Could you check a few things on this drawing? It's one solid part, dimensions in mm from its lowest x, y, z. A direction names the side the tool comes from. Coordinates: 2 decimals unless noted, no trailing zeros. Order: outer loops, then holes, each group sorted by start corner. A loop starts at its lowest first (then second) coordinate and runs counter-clockwise, first axis right, second up. Notation, with made-up numbers: M 13,3.5 L 39,3.5 A21 cw 39,28.5 Z; hole C -37.5,-26.5 d4. An arc over 180 degrees is marked long. Answer as CSV lines item,"result". Start each with the question number.
1. If we section it at A-A (z = 7.75): List the corners of the cut face in (x, y) for me, plus the area to 3 significant figures.
2. I need wall thicknesses on line 1 along Z through (x, y) = (9, 3.5); line 2 along Z through (x, y) = (5, 2.6); line 3 along Z through (x, y) = (5, 1.2). Which ranges of each line are inside material? Lowest first, please. Write a range as from..to.
3. If we mould it in two halves opening along Z, with no side actions, what happens to the marked faces 3, 4 and 5? For each: released by +Z, released by -Z, zero draft, split by the parting line, or undercut.
4. If we section it at B-B (x = 5): List the corners of the cut face in (y, z) for me.
5. If we section it at C-C (z = 4.5): List the corners of the cut face in (x, y) for me.
6. On a 3-axis mill with a long thin cutter (end or side, diameter ignored), from which of +Z, -Z, +X, -X, +Y, -Y can I reach the whole of each face in a straight line? I mean the marked faces 1 and 2. Say none if no direction works.
7. Will these pins go through, and if not, where does the flat tip stop? pin 1 (0.8 mm diameter, centred on x = 6, z = 11, fed in from +Y); pin 2 (4 mm diameter, centred on x = 5, z = 7.75, fed in from +Y).
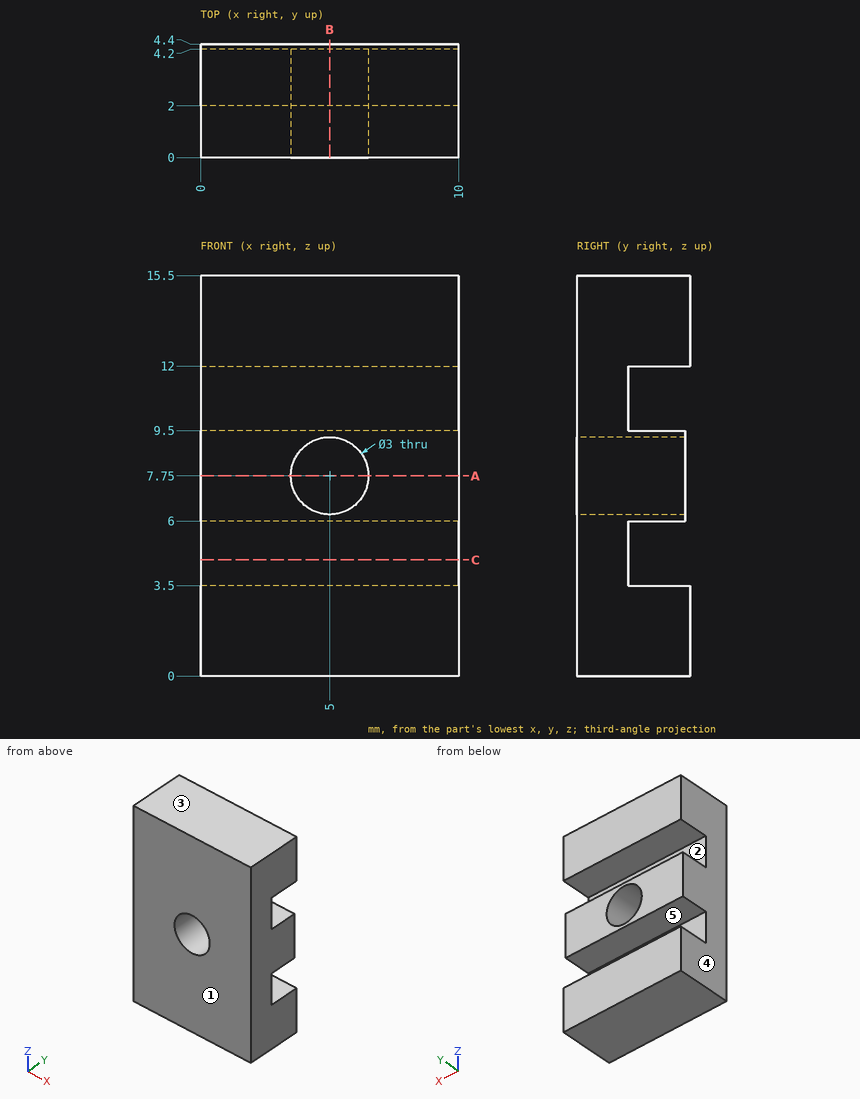
Solved:
1,outline,"M 0,0 L 3.5,0 L 3.5,4.2 L 0,4.2 Z; M 6.5,0 L 10,0 L 10,4.2 L 6.5,4.2 Z"
1,area,"29.4 mm²"
2,line 1,"0..3.5, 6..9.5, 12..15.5"
2,line 2,"0..3.5, 6..6.25, 9.25..9.5, 12..15.5"
2,line 3,"0..6.25, 9.25..15.5"
3,face 3,"released by +Z"
3,face 4,"zero draft"
3,face 5,"undercut"
4,outline,"M 0,0 L 4.4,0 L 4.4,3.5 L 2,3.5 L 2,6 L 4.2,6 L 4.2,6.25 L 0,6.25 Z; M 0,9.25 L 4.2,9.25 L 4.2,9.5 L 2,9.5 L 2,12 L 4.4,12 L 4.4,15.5 L 0,15.5 Z"
5,outline,"M 0,0 L 10,0 L 10,2 L 0,2 Z"
6,face 1,"+Z, -Z, +X, -X, -Y"
6,face 2,"+X, -X, +Y"
7,pin 1,"y = 2"
7,pin 2,"y = 4.2"
